Can you work these out from the model? Positions are in its coordinate system, mm. A direction names the side the tool comes from. Give positions to 0.01 mm unless a question says otherwise; leave off trailing zeros. Loops run counter-clockwise (first coordinate to the right, second up) from the corner with the lowest first, then second, coordinate; pieces in that order, holes last. Notation, with made-up numbers: M -34.5,-21.5 L -28.5,-21.5 A20 cw -28.5,7.5 Z; hole C 74.5,-24.75 d2. An arc over 180 degrees is marked long. Use CSV: the item, a comma, the result in double quotes.
from build123d import *

# Parameters (mm, degrees)
SKETCH1_W           = 38.1
SKETCH1_H           = 19.05
SKETCH1_W_2         = 31.75
SKETCH1_H_2         = 12.7
EXTRUDE_THIN1_DEPTH = 838.2
SKETCH2_R           = 14.2875
CUT_EXTRUDE1_DEPTH  = 840.28168841
SKETCH3_R           = 14.2875
CUT_EXTRUDE2_DEPTH  = 840.28168841


with BuildPart() as part:
    # Sketch1 → Extrude-Thin1 (new body)
    with BuildSketch(Plane(origin=(0, 0, 0), x_dir=(1, 0, 0), z_dir=(0, 1, 0))):
        with Locations((19.05, 9.525)):
            Rectangle(SKETCH1_W, SKETCH1_H)
        with Locations((19.05, 9.525)):
            Rectangle(SKETCH1_W_2, SKETCH1_H_2, mode=Mode.SUBTRACT)
    extrude(amount=EXTRUDE_THIN1_DEPTH)

    # Sketch2 → Cut-Extrude1 (cut, through all)
    with BuildSketch(Plane.XY):
        with Locations((19.05, 165.1)):
            Circle(SKETCH2_R)
    extrude(amount=-CUT_EXTRUDE1_DEPTH, mode=Mode.SUBTRACT)

    # Sketch3 → Cut-Extrude2 (cut, through all)
    with BuildSketch(Plane.XY):
        with Locations((19.05, 812.8)):
            Circle(SKETCH3_R)
    extrude(amount=-CUT_EXTRUDE2_DEPTH, mode=Mode.SUBTRACT)


solid = part.part
Q1. For faces 1 (the flat face through (34.925, 413, -9)), 2 (the flat face through (19, 413, 0)), which set-ups out of +Z, -Z, +X, -X, +Y, -Y let a thin tool reach every point of the face, with its end or its side?
Model answer:
face 1,"+Y, -Y"
face 2,"+Z, +X, -X, +Y, -Y"
Q2. I want a section at A-A, the plane z = -7.5. Please give me the cut outline in (x, y) (3 decimals).
Model answer:
outline,"M 0,0 L 3.175,0 L 3.175,838.2 L 0,838.2 Z; M 34.925,0 L 38.1,0 L 38.1,838.2 L 34.925,838.2 Z"
Q3. If we mould it in two halves opening along Z, with no side actions, what happens to faces 3 (the cylindrical face through (32.25, 159.63, -17.44)), 4 (the flat face through (19, 413, -15.875)), 5 (the flat face through (19, 413, -19.05))? For each: released by +Z, released by -Z, zero draft, split by the parting line, or undercut.
Model answer:
face 3,"zero draft"
face 4,"undercut"
face 5,"released by -Z"
Q4. I want a section at B-B, the plane x = 19.05. State how many separate pieces and enclosed holes the cut face has, then the cut area to 3 significant figures.
Model answer:
separate pieces,"6"
enclosed holes,"0"
area,"4,960 mm2"
Q5. I want a section at D-D, the plane y = 72.5. Please give me the cut outline in (x, z) (3 decimals), then the cut area to 3 significant figures.
Model answer:
outline,"M 0,-19.05 L 38.1,-19.05 L 38.1,0 L 0,0 Z; hole M 3.175,-15.875 L 34.925,-15.875 L 34.925,-3.175 L 3.175,-3.175 Z"
area,"323 mm2"
Q6. Please list where these lines run through material, in increasing order: L1, parallel to Y at x = 19.05, z = -0.75; L2, parallel to Y at x = 18, z = -17.5; L3, parallel to Z at x = 27.5, y = 82 (3 decimals). Write a range as from..to.
Model answer:
L1,"0..150.81, 179.39..798.51, 827.09..838.2"
L2,"0..150.85, 179.35..798.55, 827.05..838.2"
L3,"-19.05..-15.875, -3.175..0"
